Could you check a few things on this model? Use its own coordinates, in mm. Round coordinates to 2 decimals unless told otherwise and drop trailing zeros. Order: outer loops, then holes, each group sorted by start corner. A loop starts at its lowest first (then second) coordinate and runs counter-clockwise, first axis right, second up. Notation, with made-up numbers: (59, -21.5) - (111, -21.5) arc R18 cw to (111, -8.5) - close; hole circle Ø11 at (32.5, -18). An arc over 180 degrees is marked (long way). Use one line per item in the form item = value.
from build123d import *

# Parameters (mm, degrees)
SKETCH1_W           = 203.2
SKETCH1_H           = 203.2
BOSS_EXTRUDE1_DEPTH = 12.7
SKETCH2_R           = 9.525
SKETCH2_R_2         = 3.175
CUT_EXTRUDE1_DEPTH  = 145.244271983


with BuildPart() as part:
    # Sketch1 → Boss-Extrude1 (new body)
    with BuildSketch(Plane.XY):
        Rectangle(SKETCH1_W, SKETCH1_H)
    extrude(amount=BOSS_EXTRUDE1_DEPTH)

    # Sketch2 → Cut-Extrude1 (cut, through all)
    with BuildSketch(Plane.XY.offset(12.7)):
        Circle(SKETCH2_R)
        with Locations((39.497, 0)):
            Circle(SKETCH2_R_2)
        with Locations((-39.497, 0)):
            Circle(SKETCH2_R_2)
    extrude(amount=-CUT_EXTRUDE1_DEPTH, mode=Mode.SUBTRACT)


solid = part.part
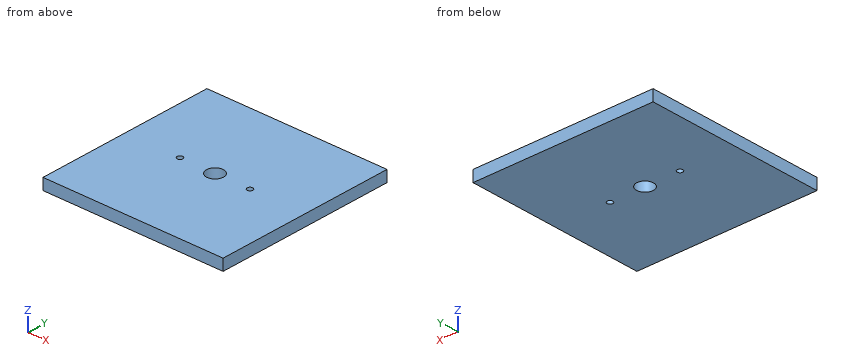
Item 1: Imagine slicing it at B-B on x = 0. Please give me the cut outline in (y, z) (3 decimals), plus the area to 3 significant figures.
Found:
outline = (-101.6, 0) - (-9.525, 0) - (-9.525, 12.7) - (-101.6, 12.7) - close; (9.525, 0) - (101.6, 0) - (101.6, 12.7) - (9.525, 12.7) - close
area = 2,340 mm2
Item 2: Imagine slicing it at A-A on y = 0. Please give me the cut outline in (x, z) (3 decimals), plus the area to 3 significant figures.
Found:
outline = (-101.6, 0) - (-42.672, 0) - (-42.672, 12.7) - (-101.6, 12.7) - close; (-36.322, 0) - (-9.525, 0) - (-9.525, 12.7) - (-36.322, 12.7) - close; (9.525, 0) - (36.322, 0) - (36.322, 12.7) - (9.525, 12.7) - close; (42.672, 0) - (101.6, 0) - (101.6, 12.7) - (42.672, 12.7) - close
area = 2,180 mm2
Item 3: Will this pin go through, and if not, where does the flat tip stop? P1, Ø5, axis at x = -39.497, y = 0, coming from the +Z side.
Found:
P1 = through
Item 4: I need wall thicknesses on L1, parallel to Y at x = 0, z = 4.75 (3 decimals); L2, parallel to X at y = 5.5, z = 10.75. Which ranges of each line are inside material? Lowest first, please.
Found:
L1 = -101.6 to -9.525, 9.525 to 101.6
L2 = -101.6 to -7.78, 7.78 to 101.6
